Part model, mm, in its own coordinate system. A direction names the side the tool comes from. Round coordinates to 2 decimals unless told otherwise and drop trailing zeros. Write each loop counter-clockwise with the first axis right and the second up, starting at its lowest first coordinate (ties: lowest second). Pieces come first, ordered by that corner, then holes. Notation, with made-up numbers: M -39,81 L -32,81 A16 ccw -32,97 Z; hole C 18.5,58.25 d11. An arc over 180 degrees is marked long. One line per question, with ' | ' between items. Start each with the question number.
1) Saw through at B-B (z = 16.5). List the corners of the cut face in (x, y), plus the area to 3 significant figures.
2) Mould opens along Z. For faces 1 (the face through (-4, -38, 39.411)), 2 (the face through (-6, -38, -13.071)), 3 (the face through (-52, -38, -5.619)), 4 (the face through (-6, 0, 6)) say: pulls with the +Z half, pulls with the -Z half, needs draft (parallel to the pull), parting line crosses it, or undercut.
3) Tool access for faces 5 (the face through (-6, -25.4, -38)), 6 (the face through (-6, -25.4, 58)), 7 (the face through (-6, -38, 32.055)): list every direction of +Z, -Z, +X, -X, +Y, -Y with a clear straight run to the whole face (end or side of a thin tool).
4) Saw through at C-C (x = -71.5). List the corners of the cut face in (y, z), plus the area to 3 significant figures.
5) Drop flat-ended pins along their axis: pin 1 Ø8 at (x, y) = (39.5, -34) entering from +Z; pin 2 Ø5 at (x, z) = (-24.5, 31) entering from +Y; pin 3 Ø12.5 at (x, y) = (11, -34) entering from -Z; pin 4 Ø3 at (y, z) = (-36.5, 14.5) entering from -X. Give the stop position or say it passes through.
6) Saw through at A-A (y = -32). List the corners of the cut face in (x, z).
7) Saw through at D-D (x = 43). List the corners of the cut face in (y, z), plus the area to 3 significant figures.
8) Wall check: probe 1 along Z at (x, y) = (-41, -28); probe 2 along Z at (x, y) = (-7.5, -26); probe 3 along Y at (x, z) = (-60, 55). Give the ranges that are in metal, low to high. Write a range as [from, to].
```python
from build123d import *

# Parameters (mm, degrees)
F0_R     = 81.8455494857
F1_DEPTH = 25.4
F3_DEPTH = 25.4


with BuildPart() as f1:
    # F0 (on Front) → F1 (new body)
    with BuildSketch(Plane.XZ):
        with Locations((-4.8047169112, 4.4472948648)):
            Circle(F0_R)
    extrude(amount=F1_DEPTH)

    # F2 (on face) → F3 (join)
    with BuildSketch(Plane.XZ.offset(25.4)):
        with BuildLine():
            ThreePointArc((-10.0211519488, -5.6191812157), (0.0460571122, 1.0869034824), (3.9396910589, 12.539409101))
            ThreePointArc((3.9396910589, 12.539409101), (-26.3024943623, 27.4354549568), (-19.6788255386, -5.6191812157))
            Line((-19.6788255386, -5.6191812157), (-10.0211519488, -5.6191812157))
        make_face()
        with BuildLine():
            Line((-10.0211519488, -5.6191812157), (-19.6788255386, -5.6191812157))
            ThreePointArc((-19.6788255386, -5.6191812157), (-14.8499887437, -6.2502707016), (-10.0211519488, -5.6191812157))
        make_face()
        with BuildLine():
            ThreePointArc((-78.8063776433, 39.4108212817), (-80.4193323461, 35.7701922921), (-81.8533073255, 32.0554220338))
            Line((-81.8533073255, 32.0554220338), (72.2438735032, 32.0554220338))
            ThreePointArc((72.2438735032, 32.0554220338), (70.8098985238, 35.7701922921), (69.1969438209, 39.4108212817))
            Line((69.1969438209, 39.4108212817), (-78.8063776433, 39.4108212817))
        make_face()
        with BuildLine():
            Line((-19.6788255386, -5.6191812157), (-86.0288514399, -5.6191812157))
            ThreePointArc((-86.0288514399, -5.6191812157), (-85.4772635025, -9.3597394685), (-84.7535081589, -13.0708314233))
            Line((-84.7535081589, -13.0708314233), (75.1440743365, -13.0708314233))
            ThreePointArc((75.1440743365, -13.0708314233), (75.8678296802, -9.3597394685), (76.4194176175, -5.6191812157))
            Line((76.4194176175, -5.6191812157), (-10.0211519488, -5.6191812157))
            ThreePointArc((-10.0211519488, -5.6191812157), (-14.8499887437, -6.2502707016), (-19.6788255386, -5.6191812157))
        make_face()
    extrude(amount=F3_DEPTH)


solid = f1.part
```
Answer key:
1) outline: M -85.76,-25.4 L -33.22,-25.4 L -33.22,-50.8 L 3.52,-50.8 L 3.52,-25.4 L 76.15,-25.4 L 76.15,0 L -85.76,0 Z | area: 5,050 mm2
2) face 1: pulls with the +Z half | face 2: pulls with the -Z half | face 3: undercut | face 4: needs draft
3) face 5: -Z, +X, -X, -Y | face 6: +Z, +X, -X, -Y | face 7: +X, -X, -Y
4) outline: M -50.8,-13.07 L -25.4,-13.07 L -25.4,-42.99 L 0,-42.99 L 0,51.89 L -25.4,51.89 L -25.4,39.41 L -50.8,39.41 L -50.8,32.06 L -25.4,32.06 L -25.4,-5.62 L -50.8,-5.62 Z | area: 2,790 mm2
5) pin 1: stops at z = 39.41 | pin 2: stops at y = 0 | pin 3: stops at z = -13.07 | pin 4: stops at x = -33.63
6) outline: M -86.03,-5.62 A81.85 ccw -84.75,-13.07 L 75.14,-13.07 A81.85 ccw 76.42,-5.62 L -10.02,-5.62 A18.79 ccw long -19.68,-5.62 Z; M -81.85,32.06 L 72.24,32.06 A81.85 ccw 69.2,39.41 L -78.81,39.41 A81.85 ccw Z
7) outline: M -50.8,-13.07 L -25.4,-13.07 L -25.4,-61.99 L 0,-61.99 L 0,70.88 L -25.4,70.88 L -25.4,39.41 L -50.8,39.41 L -50.8,32.06 L -25.4,32.06 L -25.4,-5.62 L -50.8,-5.62 Z | area: 3,750 mm2
8) probe 1: z = [-13.07, -5.62], [32.06, 39.41] | probe 2: z = [-13.07, -5.62], [-4.75, 29.83], [32.06, 39.41] | probe 3: y = [-25.4, 0]
